from build123d import *

# Parameters (mm, degrees)
F0_R            = 76.2
F0_R_2          = 14.1605
F1_DEPTH        = 3.175
F2_R            = 2.3622
F3_DEPTH        = 3.176
F3_COPIES_COUNT = 6


# Not quite as in the source:
# - a pattern or mirror of a feature is missing from the dataset's text; its kind, count and spacing are read off the source's solid


with BuildPart() as f1:
    # F0 (on Top) → F1 (new body)
    with BuildSketch(Plane.XY):
        Circle(F0_R)
        Circle(F0_R_2, mode=Mode.SUBTRACT)
    extrude(amount=F1_DEPTH)

    # F2 (on face) → F3 (cut, through all)
    with BuildSketch(Plane.XY.offset(3.175)):
        with Locations((0, 23.8125)):
            Circle(F2_R)
        with Locations((25.4, 43.9940905122)):
            Circle(F2_R)
    f3 = extrude(amount=-F3_DEPTH, mode=Mode.SUBTRACT)

    # F3_copies: F3 ×6 about axis
    f3_copies_axis = Axis((0, 0, 0), (0, 0, 1))
    for i in range(1, F3_COPIES_COUNT):
        add(f3.rotate(f3_copies_axis, i * 360 / F3_COPIES_COUNT), mode=Mode.SUBTRACT)


solid = f1.part
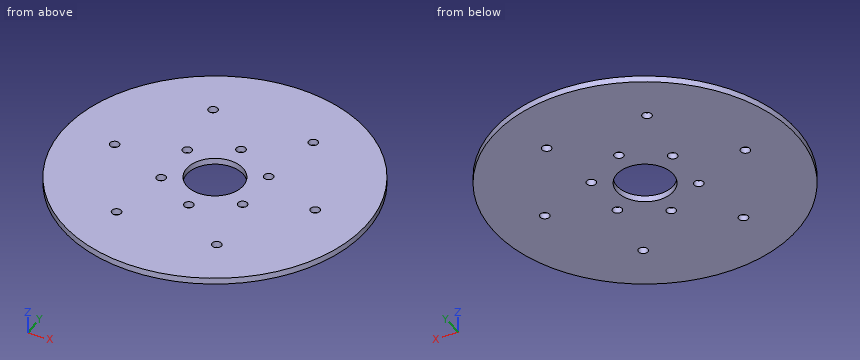
Source: CAD feature listing. Evaluate the final solid. Frame: model axes, mm. Coordinates: 2 decimals unless noted, no trailing zeros. Order: outer loops, then holes, each group sorted by start corner. A loop starts at its lowest first (then second) coordinate and runs counter-clockwise, first axis right, second up.
Item 1: Cut plane D-D (x = 16). Return loops of the section in (y, z) (3 decimals).
Output values:
outline: (-74.501, 0) - (74.501, 0) - (74.501, 3.175) - (-74.501, 3.175) - close
Item 2: Cut plane C-C (z = 2.25). Count the separate pieces of the cut face and the enclosed holes in it, plus the area to 3 significant figures.
Output values:
separate pieces: 1
enclosed holes: 13
area: 17,400 mm2
Item 3: Cut plane A-A (y = 0). Return loops of the section in (x, z) (1 decimal).
Output values:
outline: (-76.2, 0) - (-53.2, 0) - (-53.2, 3.2) - (-76.2, 3.2) - close; (-48.4, 0) - (-14.2, 0) - (-14.2, 3.2) - (-48.4, 3.2) - close; (14.2, 0) - (48.4, 0) - (48.4, 3.2) - (14.2, 3.2) - close; (53.2, 0) - (76.2, 0) - (76.2, 3.2) - (53.2, 3.2) - close
Item 4: Material intervals for line 1 (Y direction, x = 0, z = 1.55); line 2 (X direction, y = -46, z = 0.2); line 3 (Y direction, x = 25.4, z = 2.4), sorted ascending.
Output values:
line 1: y = -76.2 to -26.17, -21.45 to -14.16, 14.16 to 21.45, 26.17 to 76.2
line 2: x = -60.75 to -26.65, -24.15 to 24.15, 26.65 to 60.75
line 3: y = -71.84 to -46.36, -41.63 to 41.63, 46.36 to 71.84
Item 5: Cut plane B-B (x = 0). Return loops of the section in (y, z) (1 decimal).
Output values:
outline: (-76.2, 0) - (-26.2, 0) - (-26.2, 3.2) - (-76.2, 3.2) - close; (-21.5, 0) - (-14.2, 0) - (-14.2, 3.2) - (-21.5, 3.2) - close; (14.2, 0) - (21.5, 0) - (21.5, 3.2) - (14.2, 3.2) - close; (26.2, 0) - (76.2, 0) - (76.2, 3.2) - (26.2, 3.2) - close
